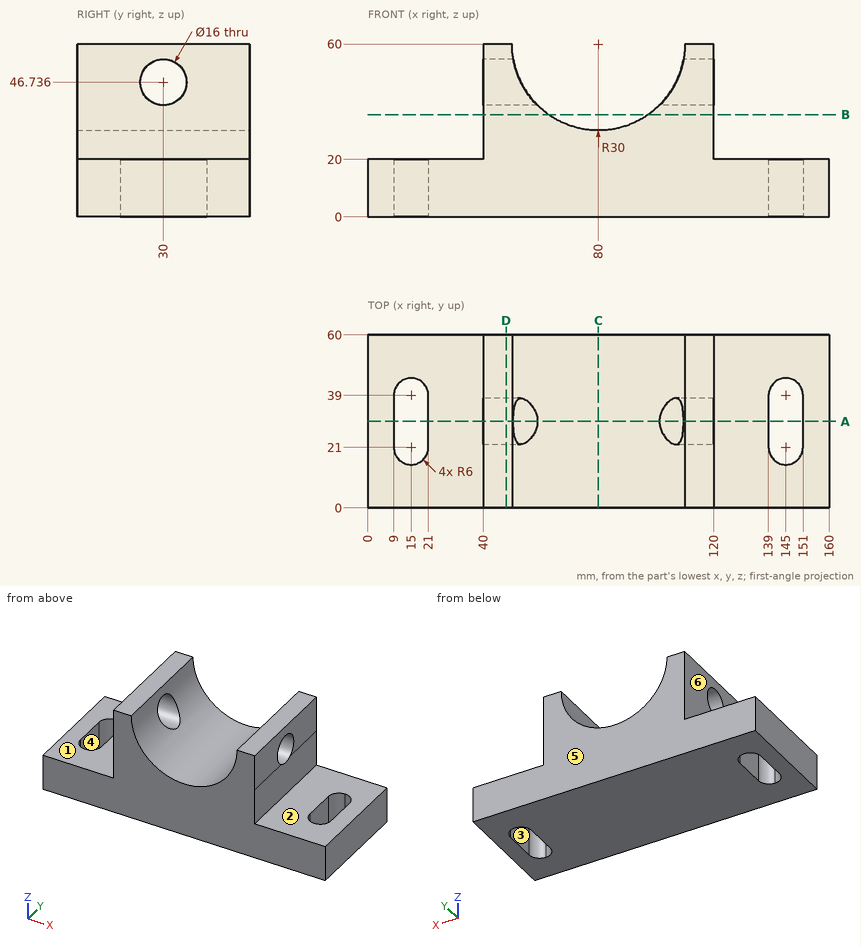
Answer from the drawing. Dimensions are ordinates in mm from the lowest x, y and z of the part. A direction names the side the tool comes from. Round coordinates to 2 decimals unless told otherwise and drop trailing zeros. Order: outer loops, then holes, each group sorted by start corner. A loop starts at its lowest first (then second) coordinate and runs counter-clockwise, first axis right, second up.
1) The mould has two halves that part along Y. Classify the marked faces 4, 5 and 6: released by +Y, released by -Y, zero draft, split by the parting line, or undercut.
2) Flat-ended cylindrical pins translate along their axes: pin 1 (13 mm diameter, centred on y = 30, z = 46.74, fed in from +X); pin 2 (21 mm diameter, centred on y = 30, z = 46.74, fed in from -X); pin 3 (10 mm diameter, centred on y = 18, z = 49.5, fed in from +X); pin 4 (12 mm diameter, centred on x = 146.5, y = 18, fed in from +Z). Find the tip coordinate at first contact, or state that the pin passes through.
3) The part is cut by section A-A on y = 30. Write down the section's boundary in (x, z), plus the area to 3 significant figures.
4) The part is cut by section D-D on x = 48. Write down the section's boundary in (y, z).
5) Straight lines are drawn through the part: L1, parallel to X at y = 24.5, z = 7; L2, parallel to Z at x = 45, y = 30; L3, parallel to X at y = 43, z = 5.5. For each, find the intervals that lie inside material, in ascending order.
6) The part is cut by section B-B on z = 35.5. Write down the section's boundary in (x, y), plus the area to 3 significant figures.
7) For the marked faces 1, 2 and 3, determine the directions among +Z, -Z, +X, -X, +Y, -Y from which every point of the face is accessible in a straight line to the end or side of a thin tool.
8) The part is cut by section C-C on x = 80. Write down the section's boundary in (y, z), plus the area to 3 significant figures.
Resolved:
1. face 4: undercut
1. face 5: released by +Y
1. face 6: zero draft
2. pin 1: passes through
2. pin 2: stops at x = 40
2. pin 3: stops at x = 120
2. pin 4: stops at z = 20
3. outline: (0, 0) - (9, 0) - (9, 20) - (0, 20) - close; (21, 0) - (139, 0) - (139, 20) - (120, 20) - (120, 38.74) - (101.16, 38.74) arc R30 cw to (58.84, 38.74) - (40, 38.74) - (40, 20) - (21, 20) - close; (40, 54.74) - (50.47, 54.74) arc R30 cw to (50, 60) - (40, 60) - close; (109.53, 54.74) - (120, 54.74) - (120, 60) - (110, 60) arc R30 cw to start; (151, 0) - (160, 0) - (160, 20) - (151, 20) - close
3. area: 4,070 mm2
4. outline: (0, 0) - (60, 0) - (60, 60) - (0, 60) - close; hole circle Ø16 at (30, 46.74)
5. L1: x = 0 to 9, 21 to 139, 151 to 160
5. L2: z = 0 to 38.74, 54.74 to 60
5. L3: x = 0 to 10.53, 19.47 to 140.53, 149.47 to 160
6. outline: (40, 0) - (62.69, 0) - (62.69, 60) - (40, 60) - close; (97.31, 0) - (120, 0) - (120, 60) - (97.31, 60) - close
6. area: 2,720 mm2
7. face 1: +Z, -X, +Y, -Y
7. face 2: +Z, +X, +Y, -Y
7. face 3: +Z, -Z
8. outline: (0, 0) - (60, 0) - (60, 30) - (0, 30) - close
8. area: 1,800 mm2
